```python
from build123d import *

# Parameters (mm, degrees)
F1_DEPTH = 25.4
F3_DEPTH = 50.801
F5_DEPTH = 13.394231155
F7_DEPTH = 15.3907378061


with BuildPart() as f1:
    # F0 (on Front) → F1 (new body)
    with BuildSketch(Plane.XZ):
        Polygon((-30.3635369193, 15.3897378061), (-30.3635369193, 0), (45.8364630807, 0), (45.8364630807, 13.393231155), (20.4364630807, 13.393231155), (20.4364630807, 47.1397378061), (-4.9635369193, 47.1397378061), (-4.9635369193, 15.3897378061), align=None)
    extrude(amount=F1_DEPTH)

    # F2 (on face) → F3 (cut, through all)
    with BuildSketch(Plane.YZ.offset(20.4364630807)):
        with BuildLine():
            Line((-19.05, 34.4397378061), (-6.35, 34.4397378061))
            ThreePointArc((-6.35, 34.4397378061), (-12.7, 40.7897378061), (-19.05, 34.4397378061))
        make_face()
        with BuildLine():
            ThreePointArc((-25.4, 34.4397378061), (-21.6802561211, 43.4199939272), (-12.7, 47.1397378061))
            Line((-12.7, 47.1397378061), (-25.4, 47.1397378061))
            Line((-25.4, 47.1397378061), (-25.4, 34.4397378061))
        make_face()
        with BuildLine():
            ThreePointArc((-12.7, 47.1397378061), (-3.7197438789, 43.4199939272), (0, 34.4397378061))
            Line((0, 34.4397378061), (0, 47.1397378061))
            Line((0, 47.1397378061), (-12.7, 47.1397378061))
        make_face()
        with BuildLine():
            ThreePointArc((-19.05, 34.4397378061), (-12.7, 28.0897378061), (-6.35, 34.4397378061))
            Line((-6.35, 34.4397378061), (-19.05, 34.4397378061))
        make_face()
    extrude(amount=-F3_DEPTH, mode=Mode.SUBTRACT)

    # F4 (on face) → F5 (cut, through all)
    with BuildSketch(Plane.XY.offset(13.393231155)):
        with BuildLine():
            ThreePointArc((39.4864630807, -12.7), (37.6265911412, -8.2098719395), (33.1364630807, -6.35))
            Line((33.1364630807, -6.35), (33.1364630807, -19.05))
            ThreePointArc((33.1364630807, -19.05), (37.6265911412, -17.1901280605), (39.4864630807, -12.7))
        make_face()
        with BuildLine():
            Line((33.1364630807, -19.05), (33.1364630807, -6.35))
            ThreePointArc((33.1364630807, -6.35), (26.7864630807, -12.7), (33.1364630807, -19.05))
        make_face()
        with BuildLine():
            Line((45.8364630807, 0), (33.33389133, 0))
            ThreePointArc((33.33389133, 0), (41.6741864681, -3.2088005425), (45.8364630807, -11.1165421488))
            Line((45.8364630807, -11.1165421488), (45.8364630807, 0))
        make_face()
        with BuildLine():
            ThreePointArc((45.8364630807, -14.2834578512), (45.9355608404, -12.7), (45.8364630807, -11.1165421488))
            Line((45.8364630807, -11.1165421488), (45.8364630807, -14.2834578512))
        make_face()
        with BuildLine():
            Line((45.8364630807, -25.4), (45.8364630807, -14.2834578512))
            ThreePointArc((45.8364630807, -14.2834578512), (41.6741864681, -22.1911994575), (33.33389133, -25.4))
            Line((33.33389133, -25.4), (45.8364630807, -25.4))
        make_face()
    extrude(amount=-F5_DEPTH, mode=Mode.SUBTRACT)

    # F6 (on face) → F7 (cut, through all)
    with BuildSketch(Plane.XY.offset(15.3897378061)):
        with BuildLine():
            ThreePointArc((-11.3135369193, -12.7), (-13.1734088588, -8.2098719395), (-17.6635369193, -6.35))
            Line((-17.6635369193, -6.35), (-17.6635369193, -19.05))
            ThreePointArc((-17.6635369193, -19.05), (-13.1734088588, -17.1901280605), (-11.3135369193, -12.7))
        make_face()
        with BuildLine():
            Line((-17.6635369193, -19.05), (-17.6635369193, -6.35))
            ThreePointArc((-17.6635369193, -6.35), (-24.0135369193, -12.7), (-17.6635369193, -19.05))
        make_face()
        with BuildLine():
            ThreePointArc((-30.3635369193, -11.1468519042), (-26.2075067106, -3.2177300877), (-17.8534793608, 0))
            Line((-17.8534793608, 0), (-30.3635369193, 0))
            Line((-30.3635369193, 0), (-30.3635369193, -11.1468519042))
        make_face()
        with BuildLine():
            Line((-30.3635369193, -14.2531480958), (-30.3635369193, -11.1468519042))
            ThreePointArc((-30.3635369193, -11.1468519042), (-30.4588632348, -12.7), (-30.3635369193, -14.2531480958))
        make_face()
        with BuildLine():
            ThreePointArc((-17.8534793608, -25.4), (-26.2075067106, -22.1822699123), (-30.3635369193, -14.2531480958))
            Line((-30.3635369193, -14.2531480958), (-30.3635369193, -25.4))
            Line((-30.3635369193, -25.4), (-17.8534793608, -25.4))
        make_face()
    extrude(amount=-F7_DEPTH, mode=Mode.SUBTRACT)


solid = f1.part
```
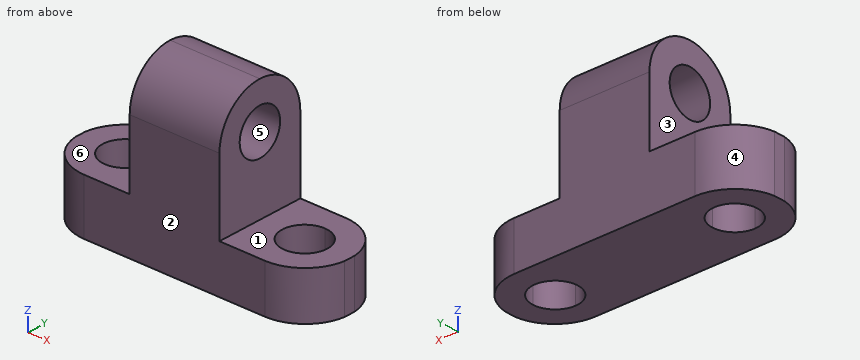
The model under review builds one solid part; all positions refer to its coordinate system, in mm. Face numbers are marked on the shaded views. A direction names the side the tool comes from. Round coordinates to 2 decimals unless told otherwise and drop trailing zeros. Loops run counter-clockwise (first coordinate to the right, second up) from the corner with the lowest first, then second, coordinate; pieces in that order, holes last. Notation, with made-up numbers: (84.25, 4) - (118.25, 4) arc R31 ccw to (118.25, 38) - close; hole circle Ø8 at (87.5, 53.25). An arc over 180 degrees is marked (long way). Use a Markdown table: item, result. Add a question column.
Q1. For probe 1 along Z at (x, y) = (14.75, -12.7); probe 2 along X at (y, z) = (-7.75, 5); probe 3 along X at (y, z) = (-9.5, 12.5), list the stretches that pass through material, from the lowest coordinate up.
Q2. Add section C-C (z = 37). State the section outline as (x, y) points.
Q3. Machinability: for the marked faces 1, 2 and 3, which of the approach directions +Z, -Z, +X, -X, +Y, -Y give a long, thin tool a straight path to every point of the face, cutting with its end or side? Answer none if there is none.
Q4. Insertion check: pin 1 Ø3 at (y, z) = (-6, 22) entering from -X; pin 2 Ø12.5 at (x, y) = (38, -13) entering from +Z. Each pin has a flat end and moves straight along its axis. Give the tip position at first contact, or say it passes through.
Q5. Add section A-A (z = 9). State the section outline as (x, y) points.
Q6. Add section B-B (x = 34.5). State the section outline as (y, z) points, plus the area to 3 significant figures.
Q7. The part is to be moulded in two halves that separate along Z. For the marked faces 4, 5 and 6, say which applies: pulls with the +Z half, pulls with the -Z half, needs draft (parallel to the pull), parting line crosses it, or undercut.
Q8. Add section D-D (y = -17). State the section outline as (x, z) points, plus the area to 3 significant figures.
Worked answers:
| question | item | result |
|---|---|---|
| 1 | probe 1 | 0 to 28.09, 40.79 to 47.14 |
| 1 | probe 2 | -29.45 to -21.64, -13.69 to 29.16, 37.11 to 44.93 |
| 1 | probe 3 | -30.05 to -23.15, -12.18 to 27.65, 38.62 to 45.53 |
| 2 | outline | (-4.96, -25.14) - (20.44, -25.14) - (20.44, -18.51) - (-4.96, -18.51) - close; (-4.96, -6.89) - (20.44, -6.89) - (20.44, -0.26) - (-4.96, -0.26) - close |
| 3 | face 1 | +Z, +X, +Y, -Y |
| 3 | face 2 | +Z, -Z, +X, -X, -Y |
| 3 | face 3 | +Z, -X, +Y, -Y |
| 4 | pin 1 | x = -4.96 |
| 4 | pin 2 | z = 13.39 |
| 5 | outline | (-30.36, -14.25) arc R12.7 ccw to (-17.85, -25.4) - (33.33, -25.4) arc R12.7 ccw to (45.84, -14.28) - (45.84, -11.12) arc R12.7 ccw to (33.33, 0) - (-17.85, 0) arc R12.7 ccw to (-30.36, -11.15) - close; hole circle Ø12.7 at (-17.66, -12.7); hole circle Ø12.7 at (33.14, -12.7) |
| 6 | outline | (-25.34, 0) - (-18.9, 0) - (-18.9, 13.39) - (-25.34, 13.39) - close; (-6.5, 0) - (-0.06, 0) - (-0.06, 13.39) - (-6.5, 13.39) - close |
| 6 | area | 172 mm² |
| 7 | face 4 | needs draft |
| 7 | face 5 | undercut |
| 7 | face 6 | pulls with the +Z half |
| 8 | outline | (-29.71, 0) - (-22.34, 0) - (-22.34, 15.39) - (-29.71, 15.39) - close; (-12.99, 0) - (28.46, 0) - (28.46, 13.39) - (20.44, 13.39) - (20.44, 29.77) - (-4.96, 29.77) - (-4.96, 15.39) - (-12.99, 15.39) - close; (-4.96, 39.11) - (20.44, 39.11) - (20.44, 46.39) - (-4.96, 46.39) - close; (37.81, 0) - (45.19, 0) - (45.19, 13.39) - (37.81, 13.39) - close |
| 8 | area | 1,380 mm² |
